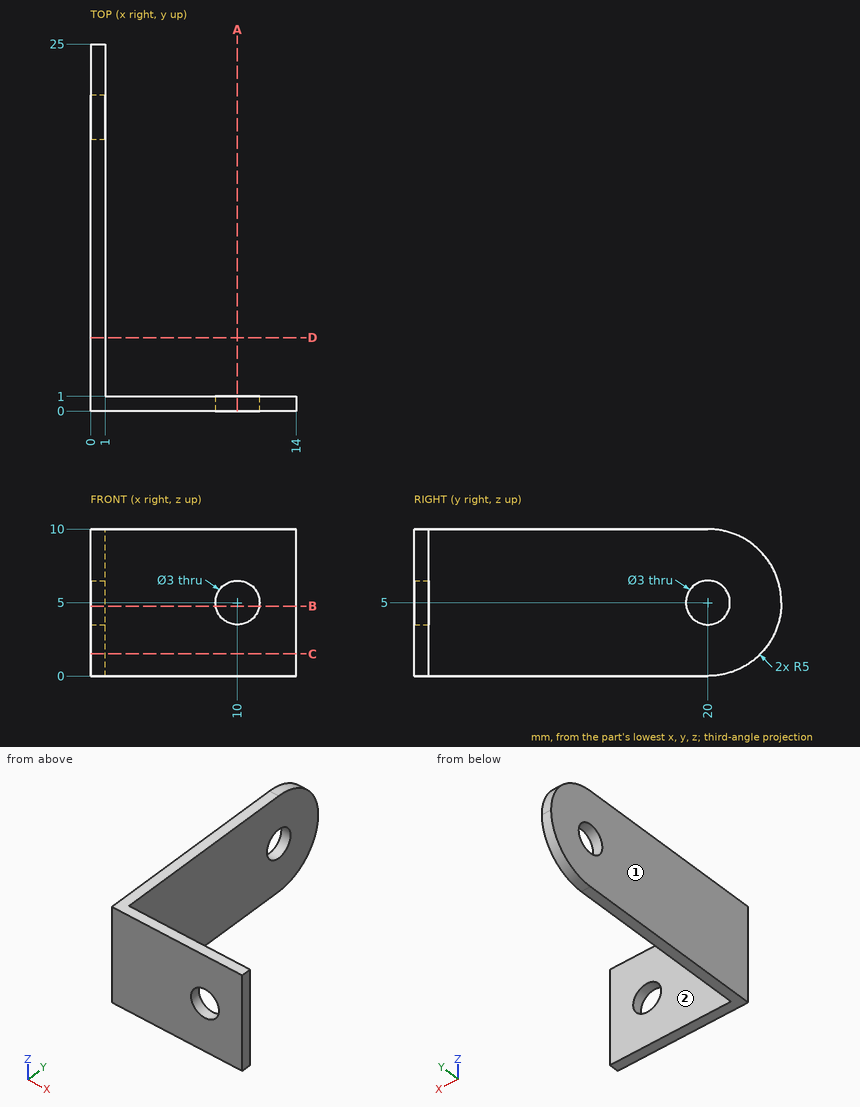
Job drawing, mm, ordinate dimensions from the low corner. One solid piece. A direction names the side the tool comes from. Give positions to 0.01 mm unless a question says otherwise; leave off trailing zeros. Order: outer loops, then holes, each group sorted by start corner. A loop starts at its lowest first (then second) coordinate and runs counter-clockwise, first axis right, second up. Notation, with made-up numbers: (75, 6.5) - (114, 6.5) arc R30 cw to (114, 32.5) - close; hole circle Ø8 at (-23.75, 21). An arc over 180 degrees is marked (long way). Return JSON: item names as keys, results as strings.
1) Cut at C-C, the plane z = 1.5. Give the cut face in (x, y).
Geometry says:
{"outline": "(0, 0) - (14, 0) - (14, 1) - (1, 1) - (1, 23.57) - (0, 23.57) - close"}
2) Cut at D-D, the plane y = 5. Give the cut face in (x, z), plus the area to 3 significant figures.
Geometry says:
{"outline": "(0, 0) - (1, 0) - (1, 10) - (0, 10) - close", "area": "10.0 mm²"}
3) Cut at A-A, the plane x = 10. Give the cut face in (y, z).
Geometry says:
{"outline": "(0, 0) - (1, 0) - (1, 3.5) - (0, 3.5) - close; (0, 6.5) - (1, 6.5) - (1, 10) - (0, 10) - close"}
4) Probe line 1 (Z direction, x = 10, y = 0.3); line 2 (Y direction, x = 8.5, z = 9). List the from-to ranges inside material, lowest first. Write a range as from..to.
Geometry says:
{"line 1": "0..3.5, 6.5..10", "line 2": "0..1"}
5) Flat gauge pins, fed straight in: P1, Ø3, axis at y = 5, z = 2.5, coming from the +X side; P2, Ø5, axis at x = 6.5, z = 7, coming from the +Y side. Where does each tip first touch, or does it go through?
Geometry says:
{"P1": "x = 1", "P2": "y = 1"}
6) 3-axis set-ups, long thin cutter, end or side, ignore diameter. For the marked faces 1 and 2: which of +Z, -Z, +X, -X, +Y, -Y reach the whole face in a straight line?
Geometry says:
{"face 1": "+Z, -Z, -X, +Y, -Y", "face 2": "+Z, -Z, +X, +Y"}
7) Cut at B-B, the plane z = 4.75. Give the cut face in (x, y), plus the area to 3 significant figures.
Geometry says:
{"outline": "(0, 0) - (8.52, 0) - (8.52, 1) - (1, 1) - (1, 18.52) - (0, 18.52) - close; (0, 21.48) - (1, 21.48) - (1, 24.99) - (0, 24.99) - close; (11.48, 0) - (14, 0) - (14, 1) - (11.48, 1) - close", "area": "32.1 mm²"}
